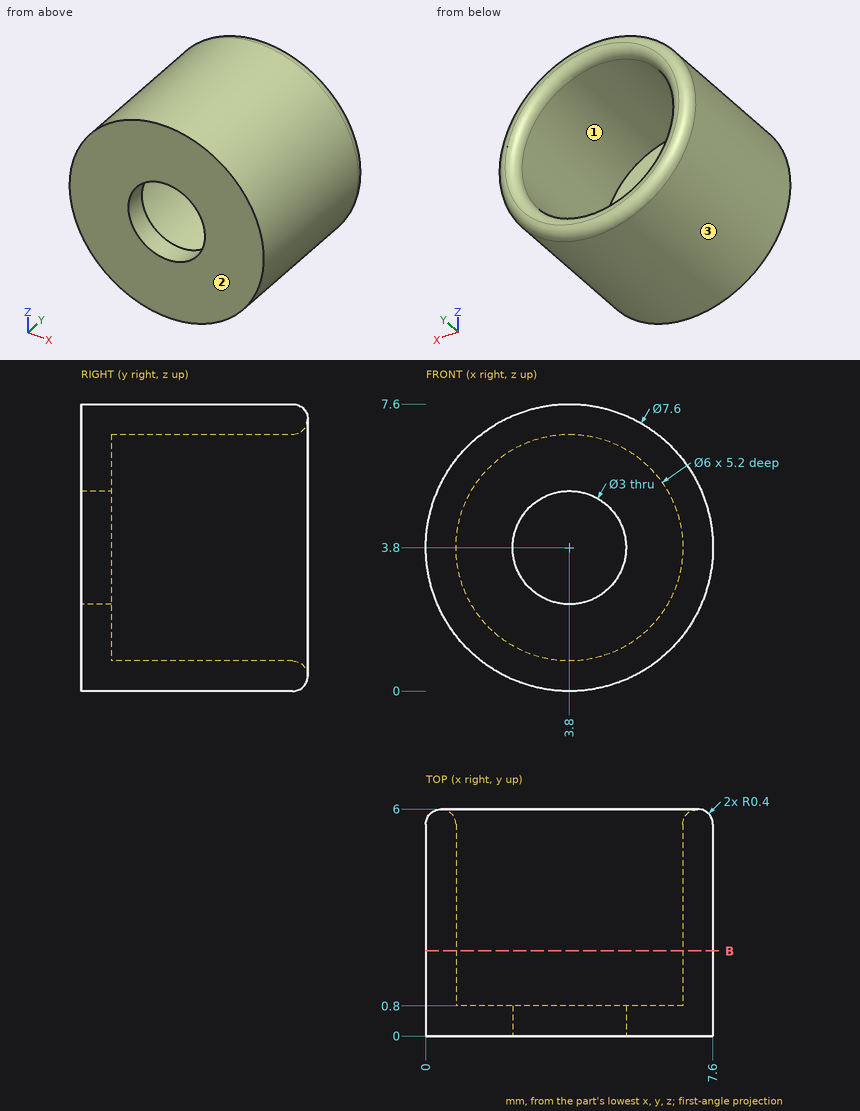
Geometry: see drawing. Coordinates: mm, zero at the bounding-box minimum. Coordinates: 2 decimals unless noted, no trailing zeros. Order: outer loops, then holes, each group sorted by start corner. A loop starts at its lowest first (then second) coordinate and runs counter-clockwise, first axis right, second up. Notation, with made-up numbers: (-15.75, -37.5) -> (37.25, -37.5) arc R17 cw to (37.25, -20.5) -> close; hole circle Ø11 at (-15.5, 49.25). An arc over 180 degrees is marked (long way). Write each question's results on one line, items separated by ' | '. Start each with the question number.
1) First-contact query: pin 1 (1.5 mm diameter, centred on y = 2.5, z = 1, fed in from -X); pin 2 (1 mm diameter, centred on y = 3, z = 4.5, fed in from +X); pin 3 (1 mm diameter, centred on x = 6.5, y = 2, fed in from -Z); pin 4 (2.5 mm diameter, centred on x = 3.8, z = 3.8, fed in from +Y). Flat tips, straight axial feed; report the tip coordinate or a pass-through.
2) Cut plane B-B, the plane y = 2.25. Output: boundary loops of the cut face in (x, z), and give its area (3 significant figures).
3) Mould query, pull axis X, two halves, no side actions, for the marked faces 1, 2 and 3. Classes: released by +X, released by -X, zero draft, split by the parting line, or undercut.
4) Material intervals for line 1 along X through (y, z) = (0.55, 3.8); line 2 along X through (y, z) = (3.15, 3.8); line 3 along Y through (x, z) = (2, 4.25), sorted ascending.
Checks:
1) pin 1: x = 0.6 | pin 2: x = 7.59 | pin 3: z = 0.7 | pin 4: through
2) outline: circle Ø7.6 at (3.8, 3.8); hole circle Ø6 at (3.8, 3.8) | area: 17.1 mm^2
3) face 1: undercut | face 2: zero draft | face 3: split by the parting line
4) line 1: 0 to 2.3, 5.3 to 7.6 | line 2: 0 to 0.8, 6.8 to 7.6 | line 3: 0 to 0.8
